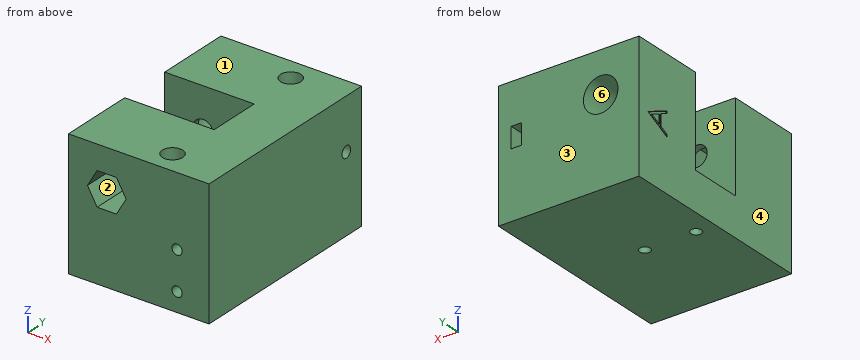
```python
from build123d import *

# Parameters (mm, degrees)
SKETCH1_W           = 55
SKETCH1_H           = 80
BOSS_EXTRUDE1_DEPTH = 50
SKETCH2_R           = 4
CUT_EXTRUDE1_DEPTH  = 110.201648339
SKETCH3_R           = 4.015
CUT_EXTRUDE2_DEPTH  = 8.03
SKETCH4_W           = 35
SKETCH4_H           = 21
CUT_EXTRUDE3_DEPTH  = 35
SKETCH8_R           = 6.75
CUT_EXTRUDE5_DEPTH  = 26.55
CUT_EXTRUDE6_DEPTH  = 26.55
SKETCH10_R          = 2
CUT_EXTRUDE7_DEPTH  = 5
SKETCH12_R          = 2.1
CUT_EXTRUDE8_DEPTH  = 104.198837203
SKETCH12_3_R        = 3.75
CUT_EXTRUDE9_DEPTH  = 4.5
SKETCH13_R          = 2.25
CUT_EXTRUDE10_DEPTH = 10
SKETCH14_W          = 4
SKETCH14_H          = 8
CUT_EXTRUDE11_DEPTH = 13
CUT_EXTRUDE12_DEPTH = 0.5


with BuildPart() as part:
    # Sketch1 → Boss-Extrude1 (new body)
    with BuildSketch(Plane.XY):
        with Locations((-27.5, 40)):
            Rectangle(SKETCH1_W, SKETCH1_H)
    extrude(amount=BOSS_EXTRUDE1_DEPTH)

    # Sketch2 → Cut-Extrude1 (cut, through all)
    with BuildSketch(Plane(origin=(0, 80, 0), x_dir=(1, 0, 0), z_dir=(0, 1, 0))):
        with Locations(Location((-40, -34, 0), (0, 0, 180))):
            Circle(SKETCH2_R)
    extrude(amount=-CUT_EXTRUDE1_DEPTH, mode=Mode.SUBTRACT)

    # Sketch3 → Cut-Extrude2 (cut)
    with BuildSketch(Plane.XY.offset(50)):
        with Locations((-21, 71)):
            Circle(SKETCH3_R)
        with Locations((-21, 9)):
            Circle(SKETCH3_R)
    extrude(amount=-CUT_EXTRUDE2_DEPTH, mode=Mode.SUBTRACT)

    # Sketch4 → Cut-Extrude3 (cut)
    with BuildSketch(Plane.XY.offset(50)):
        with Locations((-37.5, 40)):
            Rectangle(SKETCH4_W, SKETCH4_H)
    extrude(amount=-CUT_EXTRUDE3_DEPTH, mode=Mode.SUBTRACT)

    # Sketch8 → Cut-Extrude5 (cut)
    with BuildSketch(Plane(origin=(0, 80, 0), x_dir=(1, 0, 0), z_dir=(0, 1, 0))):
        with Locations(Location((-40, -34, 0), (0, 0, 180))):
            Circle(SKETCH8_R)
    extrude(amount=-CUT_EXTRUDE5_DEPTH, mode=Mode.SUBTRACT)

    # Sketch9 → Cut-Extrude6 (cut)
    with BuildSketch(Plane.XZ):
        Polygon((-32.436711474, 34), (-36.218355737, 40.55), (-43.781644263, 40.55), (-47.563288526, 34), (-43.781644263, 27.45), (-36.218355737, 27.45), align=None)
    extrude(amount=-CUT_EXTRUDE6_DEPTH, mode=Mode.SUBTRACT)

    # Sketch10 → Cut-Extrude7 (cut)
    with BuildSketch(Plane.XZ):
        with Locations(Location((-12.5, 7.5, 0), (0, 0, 270))):
            Circle(SKETCH10_R)
        with Locations(Location((-12.5, 22.5, 0), (0, 0, 270))):
            Circle(SKETCH10_R)
    extrude(amount=-CUT_EXTRUDE7_DEPTH, mode=Mode.SUBTRACT)

    # Sketch12 → Cut-Extrude8 (cut, through all)
    with BuildSketch(Plane.XY.offset(15)):
        with Locations((-47.5, 40)):
            Circle(SKETCH12_R)
        with BuildLine():
            ThreePointArc((-29.6, 40), (-27.5, 37.9), (-25.4, 40))
            Line((-25.4, 40), (-29.6, 40))
        make_face()
        with BuildLine():
            Line((-29.6, 40), (-25.4, 40))
            ThreePointArc((-25.4, 40), (-27.5, 42.1), (-29.6, 40))
        make_face()
    extrude(amount=-CUT_EXTRUDE8_DEPTH, mode=Mode.SUBTRACT)

    # Sketch12<3> → Cut-Extrude9 (cut)
    with BuildSketch(Plane.XY.offset(15)):
        with BuildLine():
            ThreePointArc((-31.25, 40), (-27.5, 36.25), (-23.75, 40))
            Line((-23.75, 40), (-25.4, 40))
            ThreePointArc((-25.4, 40), (-27.5, 37.9), (-29.6, 40))
            Line((-29.6, 40), (-31.25, 40))
        make_face()
        with BuildLine():
            Line((-25.4, 40), (-23.75, 40))
            ThreePointArc((-23.75, 40), (-27.5, 43.75), (-31.25, 40))
            Line((-31.25, 40), (-29.6, 40))
            ThreePointArc((-29.6, 40), (-27.5, 42.1), (-25.4, 40))
        make_face()
        with Locations((-47.5, 40)):
            Circle(SKETCH12_3_R)
    extrude(amount=-CUT_EXTRUDE9_DEPTH, mode=Mode.SUBTRACT)

    # Sketch13 → Cut-Extrude10 (cut)
    with BuildSketch(Plane(origin=(0, 0, 0), x_dir=(0, 0, -1), z_dir=(1, 0, 0))):
        with Locations((-30, 72)):
            Circle(SKETCH13_R)
    extrude(amount=-CUT_EXTRUDE10_DEPTH, mode=Mode.SUBTRACT)

    # Sketch14 → Cut-Extrude11 (cut)
    with BuildSketch(Plane(origin=(0, 80, 0), x_dir=(1, 0, 0), z_dir=(0, 1, 0))):
        with Locations((-7, -30)):
            Rectangle(SKETCH14_W, SKETCH14_H)
    extrude(amount=-CUT_EXTRUDE11_DEPTH, mode=Mode.SUBTRACT)

    # Sketch15 → Cut-Extrude12 (cut)
    with BuildSketch(Plane.ZY.offset(55)):
        Polygon((25.128205128, 75.25), (29.743589744, 65.25), (28.768028846, 65.25), (27.289663462, 68.455128205), (22.756410256, 68.455128205), (21.235977564, 65.25), (20.256410256, 65.25), (25, 75.25), align=None)
        Polygon((25.054086538, 73.30088141), (23.243189103, 69.480769231), (26.816907051, 69.480769231), align=None, mode=Mode.SUBTRACT)
    extrude(amount=-CUT_EXTRUDE12_DEPTH, mode=Mode.SUBTRACT)


solid = part.part
```
Geometry check sheet. Reference: the model listing, model coordinates, mm. Face numbers are marked on the shaded views. A direction names the side the tool comes from. Round coordinates to 2 decimals unless told otherwise and drop trailing zeros. Loops run counter-clockwise (first coordinate to the right, second up) from the corner with the lowest first, then second, coordinate; pieces in that order, holes last. Notation, with made-up numbers: M 39.25,83.25 L 79.25,83.25 A26 ccw 79.25,109.25 Z; hole C 4,-22 d3. An arc over 180 degrees is marked long. Return JSON: item names as keys, results as strings. Group by question number.
(1) Mould release check, pull along Z, two halves, no side actions. Record for the marked faces 1, 2 and 3: pulls with the +Z half, pulls with the -Z half, needs draft (parallel to the pull), parting line crosses it, or undercut.
(2) Section check A-A, the plane x = -40. Enter the section's corners in (y, z).
(3) Section check C-C, the plane z = 46. Enter the section's corners in (x, y) (3 decimals), and give its area (3 significant figures).
(4) Set-up check for the marked faces 4, 5 and 6: record each of +Z, -Z, +X, -X, +Y, -Y from which the full face is reachable in a straight line by a thin tool's end or side.
(5) Scan lines: line 1 along Y through (x, z) = (-27.5, 12.6); line 2 along Y through (x, z) = (-9.35, 30); line 3 along X through (y, z) = (33.5, 16). Record each from-to range of solid material in increasing order. Write a range as [from, to].
(6) Section check D-D, the plane y = 19. Enter the section's corners in (x, z).
(7) Section check B-B, the plane y = 40. Enter the section's corners in (x, z), and give its area (3 significant figures).
(8) Go/stop test with flat-tipped pins: pin 1 (6.5 mm diameter, centred on x = -40, z = 34, fed in from +Y); pin 2 (2.5 mm diameter, centred on x = -21.5, y = 72.5, fed in from +Z); pin 3 (5 mm diameter, centred on y = 38, z = 20, fed in from -X); pin 4 (7 mm diameter, centred on x = -39.5, z = 32, fed in from +Y). Record where each tip stops, or that it passes through.
Data:
{
 "1": {"face 1": "pulls with the +Z half", "face 2": "undercut", "face 3": "needs draft"},
 "2": {"outline": "M 0,0 L 80,0 L 80,27.25 L 53.45,27.25 L 53.45,30 L 50.5,30 L 50.5,15 L 29.5,15 L 29.5,30 L 26.55,30 L 26.55,27.45 L 0,27.45 Z; M 0,40.55 L 26.55,40.55 L 26.55,38 L 29.5,38 L 29.5,50 L 0,50 Z; M 50.5,38 L 53.45,38 L 53.45,40.75 L 80,40.75 L 80,50 L 50.5,50 Z"},
 "3": {"outline": "M -55,0 L 0,0 L 0,80 L -55,80 L -55,50.5 L -20,50.5 L -20,29.5 L -55,29.5 Z; hole C -21,9 d8.03; hole C -21,71 d8.03", "area": "3,560 mm²"},
 "4": {"face 4": "+Z, -Z, -X, +Y, -Y", "face 5": "+Z, -X", "face 6": "+Y"},
 "5": {"line 1": "[0, 36.25], [43.75, 80]", "line 2": "[0, 69.75], [74.25, 80]", "line 3": "[-20, 0]"},
 "6": {"outline": "M -55,0 L 0,0 L 0,50 L -55,50 Z; hole M -47.56,34 L -43.78,27.45 L -36.22,27.45 L -32.44,34 L -36.22,40.55 L -43.78,40.55 Z"},
 "7": {"outline": "M -55,0 L -49.6,0 L -49.6,10.5 L -51.25,10.5 L -51.25,15 L -55,15 Z; M -45.4,0 L -29.6,0 L -29.6,10.5 L -31.25,10.5 L -31.25,15 L -43.75,15 L -43.75,10.5 L -45.4,10.5 Z; M -25.4,0 L 0,0 L 0,50 L -20,50 L -20,15 L -23.75,15 L -23.75,10.5 L -25.4,10.5 Z", "area": "1,370 mm²"},
 "8": {"pin 1": "through", "pin 2": "z = 41.97", "pin 3": "x = -20", "pin 4": "y = 53.45"}
}
